Source: CAD feature listing. Evaluate the final solid. Frame: model axes, mm. A direction names the side the tool comes from. Give positions to 0.01 mm unless a question says otherwise; leave off trailing zeros. Order: outer loops, then holes, each group sorted by start corner. A loop starts at its lowest first (then second) coordinate and runs counter-clockwise, first axis right, second up. Notation, with made-up numbers: (52.5, 40.5) -> (75.5, 40.5) arc R29 ccw to (75.5, 64.5) -> close; hole circle Ø4 at (66, 10). An arc over 180 degrees is marked (long way). Answer in a Markdown table with one row per item.
```python
from build123d import *

# Parameters (mm, degrees)
F2_R     = 4
F3_DEPTH = 26.5


with BuildPart() as f1:
    # F0 (on Front) → F1 (revolve)
    with BuildSketch(Plane.XZ):
        with BuildLine():
            Line((0, 9), (0, -23))
            Line((0, -23), (15.151307, -23))
            Line((15.151307, -23), (15.6, -22.779377))
            Line((15.6, -22.779377), (15.6, -17.5))
            ThreePointArc((15.6, -17.5), (14.53934, -17.06066), (14.1, -16))
            Line((14.1, -16), (14.1, -10.6))
            ThreePointArc((14.1, -10.6), (13.22132, -8.47868), (11.1, -7.6))
            Line((11.1, -7.6), (8.3, 0))
            Line((8.3, 0), (8.3, 5.7))
            Line((8.3, 5.7), (5, 9))
            Line((5, 9), (0, 9))
        make_face()
    revolve(axis=Axis((0, 0, -1.903735), (0, 0, 1)))

    # F2 (on face) → F3 (cut)
    with BuildSketch(Plane.XY.offset(9)):
        Circle(F2_R)
    extrude(amount=-F3_DEPTH, mode=Mode.SUBTRACT)


solid = f1.part
```
(1) Section query A-A (x = 0). Return the cut outline in (y, z).
A:
| item | result |
|---|---|
| outline | (-15.6, -22.78) -> (-15.15, -23) -> (15.15, -23) -> (15.6, -22.78) -> (15.6, -17.5) arc R1.5 cw to (14.1, -16) -> (14.1, -10.6) arc R3 ccw to (11.1, -7.6) -> (8.3, 0) -> (8.3, 5.7) -> (5, 9) -> (4, 9) -> (4, -17.5) -> (-4, -17.5) -> (-4, 9) -> (-5, 9) -> (-8.3, 5.7) -> (-8.3, 0) -> (-11.1, -7.6) arc R3 ccw to (-14.1, -10.6) -> (-14.1, -16) arc R1.5 cw to (-15.6, -17.5) -> close |
(2) Section query C-C (z = -6). Return the cut outline in (x, y).
A:
| item | result |
|---|---|
| outline | circle Ø21.02 at (0, 0); hole circle Ø8 at (0, 0) |
(3) First-contact query: pin 1 Ø2.5 at (x, y) = (-0.5, 0) entering from +Z; pin 2 Ø5 at (x, y) = (-1, -10) entering from +Z; pin 3 Ø1.5 at (y, z) = (4, -8) entering from -X. Flat tips, straight axial feed; report the tip coordinate or a pass-through.
A:
| item | result |
|---|---|
| pin 1 | stops at z = -17.5 |
| pin 2 | stops at z = 6.45 |
| pin 3 | stops at x = -12.89 |
(4) Ray query, probe 1 along Y at (x, z) = (0, -0.25); probe 2 along Y at (x, z) = (0, -0.5); probe 3 along Z at (x, y) = (-11, 2). Return the intervals inside material, ascending.
A:
| item | result |
|---|---|
| probe 1 | y = -8.39 to -4, 4 to 8.39 |
| probe 2 | y = -8.48 to -4, 4 to 8.48 |
| probe 3 | z = -23 to -7.6 |
(5) Pull-direction query (X, two-part tool) for faces 3 (the conical face through (-4.095, -3.14, 8.84)), 4 (the cylindrical face through (-0.867, -3.905, -4.065)), 5 (the flat face through (0, 0, -23)); classes: +X half, -X half, draft (parallel to the pull), parting line (faces both ways), or undercut.
A:
| item | result |
|---|---|
| face 3 | parting line |
| face 4 | undercut |
| face 5 | draft |
(6) Access query for faces 1 (the flat face through (0, 0, -17.5)), 2 (the cylindrical face through (-11.5, 10.54, -20.1)). Directions: +Z, -Z, +X, -X, +Y, -Y. A direction counts if a zero-diameter tool reaches every point of the face in a straight line with its end or side. Return the directions, or none.
A:
| item | result |
|---|---|
| face 1 | +Z |
| face 2 | +Z, -Z |
(7) Section query B-B (z = 1.5). Return the cut outline in (x, y).
A:
| item | result |
|---|---|
| outline | circle Ø16.6 at (0, 0); hole circle Ø8 at (0, 0) |
